```python
from build123d import *

# Parameters (mm, degrees)
CYLINDER2755_R               = 2.2
CYLINDER2755_DEPTH           = 10
CYLINDER2763_R               = 1
CYLINDER2763_DEPTH           = 20
CYLINDER2763_PLACEMENT_ANGLE = 45
CYLINDER2762_R               = 1
CYLINDER2762_DEPTH           = 20
CYLINDER2760_R               = 1
CYLINDER2760_DEPTH           = 20
CYLINDER2761_R               = 1
CYLINDER2761_DEPTH           = 20
CYLINDER2761_PLACEMENT_ANGLE = 225
CYLINDER2759_R               = 1
CYLINDER2759_DEPTH           = 20
CYLINDER2759_PLACEMENT_ANGLE = 135
CYLINDER2757_R               = 1
CYLINDER2757_DEPTH           = 20
CYLINDER2757_PLACEMENT_ANGLE = 45
CYLINDER2758_R               = 1
CYLINDER2758_DEPTH           = 20
CYLINDER2756_R               = 1
CYLINDER2756_DEPTH           = 20
BOX953_W                     = 4
BOX953_H                     = 4
BOX953_DEPTH                 = 1.4
BOX953_PLACEMENT_ANGLE       = 45
BOX954_W                     = 4
BOX954_H                     = 4
BOX954_DEPTH                 = 1.4
BOX955_W                     = 4
BOX955_H                     = 4
BOX955_DEPTH                 = 1.4
BOX955_PLACEMENT_ANGLE       = 135
BOX956_W                     = 4
BOX956_H                     = 4
BOX956_DEPTH                 = 1.4
BOX957_W                     = 4
BOX957_H                     = 4
BOX957_DEPTH                 = 1.4
BOX957_PLACEMENT_ANGLE       = 225
BOX958_W                     = 4
BOX958_H                     = 4
BOX958_DEPTH                 = 1.4
BOX959_W                     = 4
BOX959_H                     = 4
BOX959_DEPTH                 = 1.4
BOX959_PLACEMENT_ANGLE       = 45
BOX952_W                     = 4
BOX952_H                     = 4
BOX952_DEPTH                 = 1.4
TORUS006_R                   = 2.2
TUBE134_R                    = 25
TUBE134_R_2                  = 21
TUBE134_DEPTH                = 14


with BuildPart() as obj1:
    # Cylinder2755 → Cylinder2755 (new body)
    with BuildSketch(Plane(origin=(20, 0, 17.5), x_dir=(1, 0, 0), z_dir=(0, 0, 1))):
        Circle(CYLINDER2755_R)
    extrude(amount=CYLINDER2755_DEPTH)


with BuildPart() as obj2:
    # Cylinder2763 → Cylinder2763 (new body)
    with BuildSketch(Plane.XY):
        Circle(CYLINDER2763_R)
    extrude(amount=CYLINDER2763_DEPTH)


with BuildPart() as obj2_1:
    # Cylinder2763 placement: moved
    add(obj2.part.moved(Location((16.26, 16.26, 8))).rotate(Axis((16.26, 16.26, 8), (0, 0, -1)), CYLINDER2763_PLACEMENT_ANGLE))


with BuildPart() as obj3:
    # Cylinder2762 → Cylinder2762 (new body)
    with BuildSketch(Plane(origin=(23, 0, 8), x_dir=(0, -1, 0), z_dir=(0, 0, 1))):
        Circle(CYLINDER2762_R)
    extrude(amount=CYLINDER2762_DEPTH)


with BuildPart() as obj4:
    # Cylinder2760 → Cylinder2760 (new body)
    with BuildSketch(Plane(origin=(0, -23, 8), x_dir=(-1, 0, 0), z_dir=(0, 0, 1))):
        Circle(CYLINDER2760_R)
    extrude(amount=CYLINDER2760_DEPTH)


with BuildPart() as obj5:
    # Cylinder2761 → Cylinder2761 (new body)
    with BuildSketch(Plane.XY):
        Circle(CYLINDER2761_R)
    extrude(amount=CYLINDER2761_DEPTH)


with BuildPart() as obj5_1:
    # Cylinder2761 placement: moved
    add(obj5.part.moved(Location((16.26, -16.26, 8))).rotate(Axis((16.26, -16.26, 8), (0, 0, 1)), CYLINDER2761_PLACEMENT_ANGLE))


with BuildPart() as obj6:
    # Cylinder2759 → Cylinder2759 (new body)
    with BuildSketch(Plane.XY):
        Circle(CYLINDER2759_R)
    extrude(amount=CYLINDER2759_DEPTH)


with BuildPart() as obj6_1:
    # Cylinder2759 placement: moved
    add(obj6.part.moved(Location((-16.26, -16.26, 8))).rotate(Axis((-16.26, -16.26, 8), (0, 0, 1)), CYLINDER2759_PLACEMENT_ANGLE))


with BuildPart() as obj7:
    # Cylinder2757 → Cylinder2757 (new body)
    with BuildSketch(Plane.XY):
        Circle(CYLINDER2757_R)
    extrude(amount=CYLINDER2757_DEPTH)


with BuildPart() as obj7_1:
    # Cylinder2757 placement: moved
    add(obj7.part.moved(Location((-16.26, 16.26, 8))).rotate(Axis((-16.26, 16.26, 8), (0, 0, 1)), CYLINDER2757_PLACEMENT_ANGLE))


with BuildPart() as obj8:
    # Cylinder2758 → Cylinder2758 (new body)
    with BuildSketch(Plane(origin=(-23, 0, 8), x_dir=(0, 1, 0), z_dir=(0, 0, 1))):
        Circle(CYLINDER2758_R)
    extrude(amount=CYLINDER2758_DEPTH)


with BuildPart() as compound1233:
    # Cylinder2756 → Cylinder2756 (new body)
    with BuildSketch(Plane(origin=(0, 23, 8), x_dir=(1, 0, 0), z_dir=(0, 0, 1))):
        Circle(CYLINDER2756_R)
    extrude(amount=CYLINDER2756_DEPTH)

    # Compound1233: union obj2, obj3, obj4, obj5, obj6, obj7, obj8
    add(obj2_1.part)
    add(obj3.part)
    add(obj4.part)
    add(obj5_1.part)
    add(obj6_1.part)
    add(obj7_1.part)
    add(obj8.part)


with BuildPart() as compound1233_1:
    # Compound1233 placement: moved
    add(compound1233.part.moved(Location((0, 0, -12))))


with BuildPart() as krychle952:
    # Box953 → Box953 (new body)
    with BuildSketch(Plane.XY):
        with Locations((2, 2)):
            Rectangle(BOX953_W, BOX953_H)
    extrude(amount=BOX953_DEPTH)


with BuildPart() as krychle952_1:
    # Box953 placement: moved
    add(krychle952.part.moved(Location((-16.263456, 13.435029, 14))).rotate(Axis((-16.263456, 13.435029, 14), (0, 0, 1)), BOX953_PLACEMENT_ANGLE))


with BuildPart() as krychle953:
    # Box954 → Box954 (new body)
    with BuildSketch(Plane(origin=(-21, -2, 14), x_dir=(0, 1, 0), z_dir=(0, 0, 1))):
        with Locations((2, 2)):
            Rectangle(BOX954_W, BOX954_H)
    extrude(amount=BOX954_DEPTH)


with BuildPart() as krychle954:
    # Box955 → Box955 (new body)
    with BuildSketch(Plane.XY):
        with Locations((2, 2)):
            Rectangle(BOX955_W, BOX955_H)
    extrude(amount=BOX955_DEPTH)


with BuildPart() as krychle954_1:
    # Box955 placement: moved
    add(krychle954.part.moved(Location((-13.435029, -16.263456, 14))).rotate(Axis((-13.435029, -16.263456, 14), (0, 0, 1)), BOX955_PLACEMENT_ANGLE))


with BuildPart() as krychle955:
    # Box956 → Box956 (new body)
    with BuildSketch(Plane(origin=(2, -21, 14), x_dir=(-1, 0, 0), z_dir=(0, 0, 1))):
        with Locations((2, 2)):
            Rectangle(BOX956_W, BOX956_H)
    extrude(amount=BOX956_DEPTH)


with BuildPart() as krychle956:
    # Box957 → Box957 (new body)
    with BuildSketch(Plane.XY):
        with Locations((2, 2)):
            Rectangle(BOX957_W, BOX957_H)
    extrude(amount=BOX957_DEPTH)


with BuildPart() as krychle956_1:
    # Box957 placement: moved
    add(krychle956.part.moved(Location((16.263456, -13.435029, 14))).rotate(Axis((16.263456, -13.435029, 14), (0, 0, 1)), BOX957_PLACEMENT_ANGLE))


with BuildPart() as krychle957:
    # Box958 → Box958 (new body)
    with BuildSketch(Plane(origin=(21, 2, 14), x_dir=(0, -1, 0), z_dir=(0, 0, 1))):
        with Locations((2, 2)):
            Rectangle(BOX958_W, BOX958_H)
    extrude(amount=BOX958_DEPTH)


with BuildPart() as krychle958:
    # Box959 → Box959 (new body)
    with BuildSketch(Plane.XY):
        with Locations((2, 2)):
            Rectangle(BOX959_W, BOX959_H)
    extrude(amount=BOX959_DEPTH)


with BuildPart() as krychle958_1:
    # Box959 placement: moved
    add(krychle958.part.moved(Location((13.435029, 16.263456, 14))).rotate(Axis((13.435029, 16.263456, 14), (0, 0, -1)), BOX959_PLACEMENT_ANGLE))


with BuildPart() as compound1234:
    # Box952 → Box952 (new body)
    with BuildSketch(Plane(origin=(-2, 21, 14), x_dir=(1, 0, 0), z_dir=(0, 0, 1))):
        with Locations((2, 2)):
            Rectangle(BOX952_W, BOX952_H)
    extrude(amount=BOX952_DEPTH)

    # Compound1234: union Krychle952, Krychle953, Krychle954, Krychle955, Krychle956, Krychle957, Krychle958
    add(krychle952_1.part)
    add(krychle953.part)
    add(krychle954_1.part)
    add(krychle955.part)
    add(krychle956_1.part)
    add(krychle957.part)
    add(krychle958_1.part)


with BuildPart() as compound1234_1:
    # Compound1234 placement: moved
    add(compound1234.part.moved(Location((0, 0, -1))))


with BuildPart() as obj9:
    # Torus006 → Torus006 (revolve)
    with BuildSketch(Plane(origin=(0, 0, 17.5), x_dir=(1, 0, 0), z_dir=(0, -1, 0))):
        with Locations((20, 0)):
            Circle(TORUS006_R)
    revolve(axis=Axis((0, 0, 17.5), (0, 0, 1)))


with BuildPart() as cut1041:
    # Tube134 → Tube134 (new body)
    with BuildSketch(Plane.XY.offset(10)):
        Circle(TUBE134_R)
        Circle(TUBE134_R_2, mode=Mode.SUBTRACT)
    extrude(amount=TUBE134_DEPTH)

    # Cut1040: cut obj9
    add(obj9.part, mode=Mode.SUBTRACT)

    # Cut1039: cut Compound1234
    add(compound1234_1.part, mode=Mode.SUBTRACT)

    # Cut1038: cut Compound1233
    add(compound1233_1.part, mode=Mode.SUBTRACT)

    # Cut1041: cut obj1
    add(obj1.part, mode=Mode.SUBTRACT)


solid = cut1041.part
```
Geometry: final body of the model. Coordinates: model frame, mm. A direction names the side the tool comes from. Round coordinates to 2 decimals unless told otherwise and drop trailing zeros. Order: outer loops, then holes, each group sorted by start corner. A loop starts at its lowest first (then second) coordinate and runs counter-clockwise, first axis right, second up. Notation, with made-up numbers: (64, -29) -> (120, -29) arc R23 cw to (120, -9) -> close; hole circle Ø7 at (48.25, 50). An arc over 180 degrees is marked (long way). Write each question's results on one line, items separated by ' | '.
Q1. Pull-direction query (Y, two-part tool) for faces 6 (the face through (-22, 0, 15)), 7 (the face through (-15, 15, 24)), 8 (the face through (20.03, 6.31, 12.73)), 9 (the face through (-17.63, -14.8, 13.69)); classes: released by +Y, released by -Y, zero draft, split by the parting line, or undercut.
Response values:
face 6: undercut | face 7: zero draft | face 8: undercut | face 9: released by -Y
Q2. Pin query (flat end, axial travel): pin 1 Ø3 at (y, z) = (3, 20) entering from -X; pin 2 Ø12 at (x, y) = (-7.5, 16) entering from -Z; pin 3 Ø4 at (x, z) = (-13, 18) entering from +Y; pin 4 Ø2 at (y, z) = (15.5, 14) entering from -X. Return the tip coordinate at first contact, or that it passes through.
Response values:
pin 1: x = -24.95 | pin 2: z = 10 | pin 3: y = 22.45 | pin 4: x = -20.37
Q3. Ray query, line 1 along X through (y, z) = (0, 12.05); line 2 along Z through (x, y) = (22.5, 1.5). Return the intervals inside material, ascending.
Response values:
line 1: -25 to -24, -22 to -21, 21 to 22, 24 to 25 | line 2: 10 to 13, 14.4 to 24
Q4. Section query B-B (z = 12.25). Count the separate pieces of the cut face and the enclosed holes in it, and give its area (3 significant figures).
Response values:
separate pieces: 1 | enclosed holes: 9 | area: 553 mm²
Q5. Access query for faces 1 (the face through (17, -15, 13)), 2 (the face through (24, 1, 13)), 3 (the face through (-16.476, 17.236, 11.479)), 4 (the face through (-2, -23, 14)), 5 (the face through (-17.63, 14.8, 13.69)). Directions: +Z, -Z, +X, -X, +Y, -Y. A direction counts if a zero-diameter tool reaches every point of the face in a straight line with its end or side. Return the directions, or none.
Response values:
face 1: none | face 2: +X | face 3: -Z | face 4: -Y | face 5: +Y
Q6. Section query C-C (z = 21). Output: boundary loops of the cut face in (x, y).
Response values:
outline: circle Ø50 at (0, 0); hole (20.9, -2.01) arc R2.2 ccw to (20.9, 2.01) arc R21 ccw (long way) to start
Q7. Section query A-A (x = 23). Output: boundary loops of the cut face in (y, z).
Response values:
outline: (-9.8, 10) -> (-1, 10) -> (-1, 13) -> (-2, 13) -> (-2, 14.4) -> (-1, 14.4) -> (-1, 16) -> (1, 16) -> (1, 14.4) -> (2, 14.4) -> (2, 13) -> (1, 13) -> (1, 10) -> (9.8, 10) -> (9.8, 24) -> (-9.8, 24) -> close
